CAD build for the part. Positions are in the model's coordinates, mm. A direction names the side the tool comes from. Round coordinates to 2 decimals unless told otherwise and drop trailing zeros. Order: outer loops, then holes, each group sorted by start corner. A loop starts at its lowest first (then second) coordinate and runs counter-clockwise, first axis right, second up. Notation, with made-up numbers: (35.5, -17) -> (39.5, -17) arc R15 ccw to (39.5, 10) -> close; hole circle Ø8 at (-27, 85). An arc over 180 degrees is marked (long way). Return JSON: item names as keys, results as strings. Group by question number.
Q1. Probe line 1 along Z through (x, y) = (3.7, -8.5); line 2 along Z through (x, y) = (-3.7, -4.5); line 3 along X through (y, z) = (3, 1.5). List the from-to ranges inside material, lowest first.
Q2. Mould opens along Z. For faces 4 (the flat face through (-4, 1.5, -3)), 5 (the cylindrical face through (-0.052, 8.199, -4.515)), 6 (the flat face through (0, 7, 4.8)) say: +Z half, -Z half, draft (parallel to the pull), parting line (faces both ways), or undercut.
Q3. Cut at B-B (z = -1). Count the separate pieces of the cut face and the enclosed holes in it, then the cut area to 3 significant figures.
Q4. Flat gauge pins, fed straight in: pin 1 (1 mm diameter, centred on x = -3.5, y = 6, fed in from -Z); pin 2 (1.5 mm diameter, centred on x = -4, y = 5.5, fed in from +Z); pin 3 (1.9 mm diameter, centred on x = 5, z = 0, fed in from +Y); pin 4 (5 mm diameter, centred on x = 3.7, z = 0, fed in from +Y). Where does each tip first touch, or does it go through?
Q5. Which spindle directions (+Z, -Z, +X, -X, +Y, -Y) get a long thin tool onto all of the face, cutting with end or side? Do faces 1 (the flat face through (-0.84, -12.08, 2.66)), 2 (the flat face through (3, -8, 3.7)), 3 (the cylindrical face through (1, -7, 0)). Say none if no direction does.
Q6. Cut at A-A (y = -10). Write the cut outline in (x, z), then the cut area to 3 significant figures.
from build123d import *

# Parameters (mm, degrees)
F0_R      = 2.8
F1_DEPTH  = 1.5
F0_R_2    = 2.425
F2_DEPTH  = 2.2
F3_R      = 2.7
F4_DEPTH  = 2.5
F5_R      = 2.7
F6_DEPTH  = 7.5
F7_R      = 3.2
F8_DEPTH  = 7
F9_R      = 1
F10_SIZE  = 0.25
F11_R     = 1.5
F12_DEPTH = 8.5


# Not quite as in the source:
# - a feature names something its author has since deleted; it is built from what else it names


with BuildPart() as f1:
    # F0 (on Front) → F1 (new body)
    with BuildSketch(Plane.XZ):
        with BuildLine():
            Line((0, 4.8), (-3.7, 4.8))
            ThreePointArc((-3.7, 4.8), (-7.0941125497, 3.3941125497), (-8.5, 0))
            ThreePointArc((-8.5, 0), (-7.0941125497, -3.3941125497), (-3.7, -4.8))
            Line((-3.7, -4.8), (0, -4.8))
            Line((0, -4.8), (3.7, -4.8))
            ThreePointArc((3.7, -4.8), (7.0941125497, -3.3941125497), (8.5, 0))
            ThreePointArc((8.5, 0), (7.0941125497, 3.3941125497), (3.7, 4.8))
            Line((3.7, 4.8), (0, 4.8))
        make_face()
        with Locations((-3.7, 0)):
            Circle(F0_R, mode=Mode.SUBTRACT)
        with Locations((3.7, 0)):
            Circle(F0_R, mode=Mode.SUBTRACT)
    extrude(amount=-F1_DEPTH)

    # F0 (on Front) → F2 (join)
    with BuildSketch(Plane.XZ):
        with BuildLine():
            Line((0, 4.8), (-3.7, 4.8))
            ThreePointArc((-3.7, 4.8), (-7.0941125497, 3.3941125497), (-8.5, 0))
            ThreePointArc((-8.5, 0), (-7.0941125497, -3.3941125497), (-3.7, -4.8))
            Line((-3.7, -4.8), (0, -4.8))
            Line((0, -4.8), (3.7, -4.8))
            ThreePointArc((3.7, -4.8), (7.0941125497, -3.3941125497), (8.5, 0))
            ThreePointArc((8.5, 0), (7.0941125497, 3.3941125497), (3.7, 4.8))
            Line((3.7, 4.8), (0, 4.8))
        make_face()
        with Locations((-3.7, 0)):
            Circle(F0_R, mode=Mode.SUBTRACT)
        with Locations((3.7, 0)):
            Circle(F0_R, mode=Mode.SUBTRACT)
        with Locations((-3.7, 0)):
            Circle(F0_R)
        with Locations((-3.7, 0)):
            Circle(F0_R_2, mode=Mode.SUBTRACT)
        with Locations((3.7, 0)):
            Circle(F0_R)
        with Locations((3.7, 0)):
            Circle(F0_R_2, mode=Mode.SUBTRACT)
    extrude(amount=F2_DEPTH)

    # F3 (on face) → F4 (join)
    with BuildSketch(Plane.XZ.offset(2.2)):
        with BuildLine():
            ThreePointArc((3.7, -4.8), (8.5, 0), (3.7, 4.8))
            Line((3.7, 4.8), (-3.7, 4.8))
            ThreePointArc((-3.7, 4.8), (-8.5, 0), (-3.7, -4.8))
            Line((-3.7, -4.8), (3.7, -4.8))
        make_face()
        with Locations((-3.7, 0)):
            Circle(F3_R, mode=Mode.SUBTRACT)
        with Locations((3.7, 0)):
            Circle(F3_R, mode=Mode.SUBTRACT)
    extrude(amount=F4_DEPTH)

    # F5 (on face) → F6 (join)
    with BuildSketch(Plane.XZ.offset(4.7)):
        with BuildLine():
            ThreePointArc((-3.7, 3.7), (-7.4, 0), (-3.7, -3.7))
            Line((-3.7, -3.7), (0, -3.7))
            Line((0, -3.7), (3.7, -3.7))
            ThreePointArc((3.7, -3.7), (7.4, 0), (3.7, 3.7))
            Line((3.7, 3.7), (1.7, 3.7))
            Line((1.7, 3.7), (0, 2))
            Line((0, 2), (-1.7, 3.7))
            Line((-1.7, 3.7), (-3.7, 3.7))
        make_face()
        with Locations((-3.7, 0)):
            Circle(F5_R, mode=Mode.SUBTRACT)
        with Locations((3.7, 0)):
            Circle(F5_R, mode=Mode.SUBTRACT)
    extrude(amount=F6_DEPTH)

    # F7 (on face) → F8 (join)
    with BuildSketch(Plane(origin=(0, 1.5, 0), x_dir=(-1, 0, 0), z_dir=(0, 1, 0))):
        with BuildLine():
            ThreePointArc((3.7, -4.8), (8.5, 0), (3.7, 4.8))
            Line((3.7, 4.8), (-3.7, 4.8))
            ThreePointArc((-3.7, 4.8), (-8.5, 0), (-3.7, -4.8))
            Line((-3.7, -4.8), (3.7, -4.8))
        make_face()
        with Locations((-3.7, 0)):
            Circle(F7_R, mode=Mode.SUBTRACT)
        with Locations((3.7, 0)):
            Circle(F7_R, mode=Mode.SUBTRACT)
    extrude(amount=F8_DEPTH)

    # F9
    f9_edges = [f1.edges().sort_by_distance(p)[0] for p in [
        (0, 8.5, 4.8),
    ]]
    fillet(f9_edges, radius=F9_R)

    # F10
    f10_edges = [f1.edges().sort_by_distance(p)[0] for p in [
        (-2.7, -12.2, 3.7),
        (-0.85, -12.2, 2.85),
        (0.85, -12.2, 2.85),
    ]]
    chamfer(f10_edges, length=F10_SIZE)

    # F11 (on Right) → F12 (cut, symmetric)
    with BuildSketch(Plane.YZ):
        with Locations((1.5, 5.8)):
            Circle(F11_R)
        with Locations((-2.5, 5.8)):
            Circle(F11_R)
        with Locations((-2.5, -5.8)):
            Circle(F11_R)
        with Locations((1.5, -5.8)):
            Circle(F11_R)
        with Locations((5.5, -5.8)):
            Circle(F11_R)
        with Locations((5.5, 5.8)):
            Circle(F11_R)
    extrude(amount=F12_DEPTH, both=True, mode=Mode.SUBTRACT)


solid = f1.part
Solution:
{
 "1": {"line 1": "z = -3.7 to -2.7, 2.7 to 3.7", "line 2": "z = -4.8 to -2.7, 2.7 to 4.8", "line 3": "x = -8.26 to -6.53, -0.87 to 0.87, 6.53 to 8.26"},
 "2": {"face 4": "undercut", "face 5": "-Z half", "face 6": "+Z half"},
 "3": {"separate pieces": "3", "enclosed holes": "0", "area": "109 mm²"},
 "4": {"pin 1": "stops at z = -4.68", "pin 2": "stops at z = 4.5", "pin 3": "passes through", "pin 4": "stops at y = 0"},
 "5": {"face 1": "+Z, -Y", "face 2": "+Z, +X, -X, -Y", "face 3": "-Y"},
 "6": {"outline": "(-3.7, -3.7) -> (3.7, -3.7) arc R3.7 ccw to (3.7, 3.7) -> (1.7, 3.7) -> (0, 2) -> (-1.7, 3.7) -> (-3.7, 3.7) arc R3.7 ccw to start; hole circle Ø5.4 at (-3.7, 0); hole circle Ø5.4 at (3.7, 0)", "area": "49.1 mm²"}
}
